Here's how the part is built. I have some questions about the finished solid (model axes, mm). Face numbers are marked on the shaded views. Round coordinates to 2 decimals unless told otherwise and drop trailing zeros. Loops run counter-clockwise (first coordinate to the right, second up) from the corner with the lowest first, then second, coordinate; pieces in that order, holes last. Notation, with made-up numbers: (83.5, -3.5) - (111.5, -3.5) arc R30 cw to (111.5, 34.5) - close; hole circle Ø7 at (36, -29). An arc over 180 degrees is marked (long way). Return JSON: item names as keys, results as strings. Group by question number.
```python
from build123d import *

# Parameters (mm, degrees)
F0_R     = 2.5
F0_R_2   = 5
F1_DEPTH = 80
F3_DEPTH = 1.5
F4_W     = 20
F4_H     = 78.5
F5_DEPTH = 1.5
F6_R     = 1.45
F7_DEPTH = 25


with BuildPart() as f1:
    # F0 (on Top) → F1 (new body)
    with BuildSketch(Plane.XY):
        with BuildLine():
            ThreePointArc((-11.5, 54.037024), (-12.481239, 51.062204), (-15.039823, 49.254987))
            ThreePointArc((-15.039823, 49.254987), (0, -51.5), (15.039823, 49.254987))
            ThreePointArc((15.039823, 49.254987), (12.481239, 51.062204), (11.5, 54.037024))
            Line((11.5, 54.037024), (11.5, 63))
            Line((11.5, 63), (-11.5, 63))
            Line((-11.5, 63), (-11.5, 54.037024))
        make_face()
        with BuildLine():
            ThreePointArc((14.128187, -47.962426), (-46.265444, -18.960715), (-23.594284, 44.082987))
            ThreePointArc((-23.594284, 44.082987), (-19.172369, 46.219688), (-14.562166, 47.912278))
            ThreePointArc((-14.562166, 47.912278), (-11.263306, 50.266106), (-10, 54.116696))
            Line((-10, 54.116696), (-10, 61.5))
            Line((-10, 61.5), (10, 61.5))
            Line((10, 61.5), (10, 54.326904))
            ThreePointArc((10, 54.326904), (11.293239, 50.435935), (14.658351, 48.093259))
            ThreePointArc((14.658351, 48.093259), (50.491326, -0.080985), (14.229822, -47.933499))
            ThreePointArc((14.229822, -47.933499), (14.179012, -47.94799), (14.128187, -47.962426))
        make_face(mode=Mode.SUBTRACT)
        with Locations((-6.25, 57.75)):
            Circle(F0_R)
        with Locations((6.25, 57.75)):
            Circle(F0_R)
        Circle(F0_R_2)
    extrude(amount=F1_DEPTH)

    # F2 (on face) → F3 (join)
    with BuildSketch(Plane(origin=(0, 0, 0), x_dir=(1, 0, 0), z_dir=(0, 0, -1))):
        with BuildLine():
            ThreePointArc((11.5, -54.037024), (12.481239, -51.062204), (15.039823, -49.254987))
            ThreePointArc((15.039823, -49.254987), (0, 51.5), (-15.039823, -49.254987))
            ThreePointArc((-15.039823, -49.254987), (-12.481239, -51.062204), (-11.5, -54.037024))
            Line((-11.5, -54.037024), (-11.5, -63))
            Line((-11.5, -63), (11.5, -63))
            Line((11.5, -63), (11.5, -54.037024))
        make_face()
    extrude(amount=F3_DEPTH)

    # F4 (on face) → F5 (cut, through all)
    with BuildSketch(Plane(origin=(0, 63, 0), x_dir=(-1, 0, 0), z_dir=(0, 1, 0))):
        with Locations((0, 39.25)):
            Rectangle(F4_W, F4_H)
    extrude(amount=-F5_DEPTH, mode=Mode.SUBTRACT)

    # F6 (on face) → F7 (cut)
    with BuildSketch(Plane.XY.offset(80)):
        Circle(F6_R)
        with Locations((-6.25, 57.75)):
            Circle(F6_R)
        with Locations((6.25, 57.75)):
            Circle(F6_R)
    extrude(amount=-F7_DEPTH, mode=Mode.SUBTRACT)


solid = f1.part
```
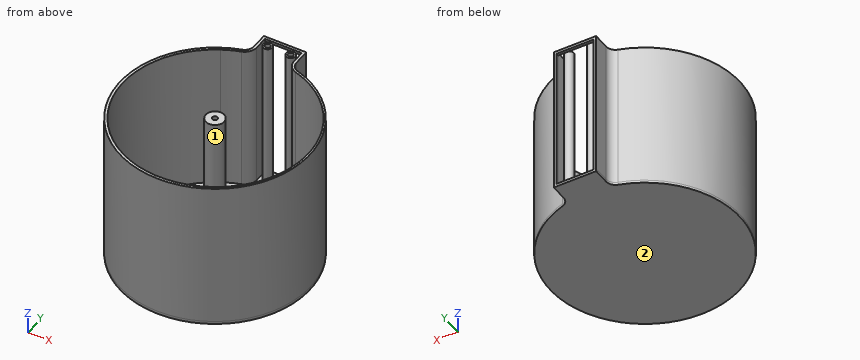
Q1. Please list where these lines run through material, in increasing order: line 1 (Y direction, x = 6, z = 67); line 2 (X direction, y = -3.5, z = 11); line 3 (X direction, y = 57, z = 67).
Q2. Will these pins go through, and if not, where does the flat tip stop? pin 1 Ø1 at (y, z) = (16, 9) entering from +X; pin 2 Ø1.5 at (x, z) = (25, 41) entering from +Y; pin 3 Ø1.7 at (x, y) = (6.25, 57.75) entering from +Z.
Q3. If we mould it in two halves opening along X, with no side actions, what happens to the marked faces 1 and 2? For each: +X half, -X half, draft (parallel to the pull), parting line (faces both ways), or undercut.
Q4. Imagine slicing it at B-B, the plane z = 21. List the corners of the cut face in (x, y) for me.
Q5. Imagine slicing it at A-A, the plane z = 66.5. List the corners of the cut face in (x, y) for me, and give its area (3 significant figures).
Q6. Imagine slicing it at C-C, the plane x = 0. List the corners of the cut face in (y, z) for me, and give its area (3 significant figures).
Q7. Imagine slicing it at D-D, the plane y = 57.75. List the corners of the cut face in (x, z) for me, and give its area (4 significant figures).
Output values:
{
 "1": {"line 1": "y = -51.15 to -49.64, 55.26 to 56.32, 59.18 to 60.24", "line 2": "x = -51.38 to -49.88, -3.57 to 3.57, 50.36 to 51.38", "line 3": "x = -11.5 to -10, -8.63 to -7.49, -5.01 to -3.87, 3.87 to 5.01, 7.49 to 8.63, 10 to 11.5"},
 "2": {"pin 1": "stops at x = 49.11", "pin 2": "stops at y = 45.43", "pin 3": "stops at z = 55"},
 "3": {"face 1": "undercut", "face 2": "draft"},
 "4": {"outline": "(-23.59, 44.08) arc R50 cw to (-14.56, 47.91) arc R6.5 ccw to (-10, 54.12) - (-10, 63) - (-11.5, 63) - (-11.5, 54.04) arc R5 cw to (-15.04, 49.25) arc R51.5 ccw (long way) to (15.04, 49.25) arc R5 cw to (11.5, 54.04) - (11.5, 63) - (10, 63) - (10, 54.33) arc R6.5 ccw to (14.66, 48.09) arc R50 cw to (14.23, -47.93) arc R48.97 cw to (14.13, -47.96) arc R50 cw to start; circle Ø5 at (-6.25, 57.75); circle Ø10 at (0, 0); circle Ø5 at (6.25, 57.75)"},
 "5": {"outline": "(-23.59, 44.08) arc R50 cw to (-14.56, 47.91) arc R6.5 ccw to (-10, 54.12) - (-10, 63) - (-11.5, 63) - (-11.5, 54.04) arc R5 cw to (-15.04, 49.25) arc R51.5 ccw (long way) to (15.04, 49.25) arc R5 cw to (11.5, 54.04) - (11.5, 63) - (10, 63) - (10, 54.33) arc R6.5 ccw to (14.66, 48.09) arc R50 cw to (14.23, -47.93) arc R48.97 cw to (14.13, -47.96) arc R50 cw to start; circle Ø5 at (-6.25, 57.75); circle Ø10 at (0, 0); circle Ø5 at (6.25, 57.75); hole circle Ø2.9 at (-6.25, 57.75); hole circle Ø2.9 at (0, 0); hole circle Ø2.9 at (6.25, 57.75)", "area": "531 mm^2"},
 "6": {"outline": "(-51.5, -1.5) - (63, -1.5) - (63, 0) - (5, 0) - (5, 80) - (1.45, 80) - (1.45, 55) - (-1.45, 55) - (-1.45, 80) - (-5, 80) - (-5, 0) - (-50, 0) - (-50, 80) - (-51.5, 80) - close; (61.5, 78.5) - (63, 78.5) - (63, 80) - (61.5, 80) - close", "area": "1,020 mm^2"},
 "7": {"outline": "(-11.5, -1.5) - (11.5, -1.5) - (11.5, 80) - (10, 80) - (10, 0) - (8.75, 0) - (8.75, 80) - (7.7, 80) - (7.7, 55) - (4.8, 55) - (4.8, 80) - (3.75, 80) - (3.75, 0) - (-3.75, 0) - (-3.75, 80) - (-4.8, 80) - (-4.8, 55) - (-7.7, 55) - (-7.7, 80) - (-8.75, 80) - (-8.75, 0) - (-10, 0) - (-10, 80) - (-11.5, 80) - close", "area": "929.5 mm^2"}
}
